from build123d import *

# Parameters (mm, degrees)
BOSS_EXTRUDE1_DEPTH           = 32
SKETCH1_3_R                   = 5
CUT_EXTRUDE1_DEPTH            = 94.618841069
CUT_EXTRUDE2_START            = -32
SKETCH2_R                     = 11.05
CUT_EXTRUDE2_DEPTH            = 5.5
M3_CLEARANCE_HOLE1_D          = 3.4
MOTOR_START                   = -5
MOTOR_POCKET_DEPTH            = 89.618841069
SKETCH6_R                     = 11
PILOT_DEPTH                   = 94.618841069
M3_CLEARANCE_HOLE2_D          = 3.4
SKETCH10_R                    = 10.35
BEARING_BORE_DEPTH            = 94.618841069
CUT_EXTRUDE6_START            = -12
CUT_EXTRUDE6_DEPTH            = 12
CUT_EXTRUDE14_START           = 3
CUT_EXTRUDE14_DEPTH           = 10
FILLET7_R                     = 5
FILLET11_R                    = 5
M3_CLEARANCE_HOLE4_D          = 3.4
CUT_EXTRUDE13_DEPTH           = 91.10972771
CUT_EXTRUDE13_DEPTH_BACK      = 3
SKETCH28_R                    = 4.7625
CUT_EXTRUDE17_DEPTH           = 45
SKETCH29_W                    = 30
SKETCH29_H                    = 10
CUT_EXTRUDE18_DEPTH           = 8.2625
CBORE_FOR_M3_SHCS1_AT_2_COUNT = 2
CBORE_FOR_M3_SHCS1_AT_2_PITCH = 25
CBORE_FOR_M3_SHCS1_AT_3_COUNT = 2
CBORE_FOR_M3_SHCS1_AT_3_PITCH = 32.015621187
CBORE_FOR_M3_SHCS1_AT_4_COUNT = 2
CBORE_FOR_M3_SHCS1_AT_4_PITCH = 20
SKETCH32_R                    = 3.25
CUT_EXTRUDE19_DEPTH           = 91.224649642


with BuildPart() as part:
    # Sketch1 → Boss-Extrude1 (new body)
    with BuildSketch(Plane(origin=(0, 0, 0), x_dir=(1, 0, 0), z_dir=(0, 1, 0))):
        with BuildLine():
            Line((0, 36.638737867), (40, -3.361262133))
            Line((40, -3.361262133), (40, -43.361262133))
            Line((40, -43.361262133), (39, -43.361262133))
            ThreePointArc((39, -43.361262133), (22.029437252, -50.390699384), (15, -67.361262133))
            Line((15, -67.361262133), (15, -78.361262133))
            Line((15, -78.361262133), (-15, -78.361262133))
            Line((-15, -78.361262133), (-15, -67.361262133))
            ThreePointArc((-15, -67.361262133), (-22.029437252, -50.390699384), (-39, -43.361262133))
            Line((-39, -43.361262133), (-40, -43.361262133))
            Line((-40, -43.361262133), (-40, -3.361262133))
            Line((-40, -3.361262133), (0, 36.638737867))
        make_face()
    extrude(amount=BOSS_EXTRUDE1_DEPTH)

    # Sketch1<3> → Cut-Extrude1 (cut, through all)
    with BuildSketch(Plane(origin=(0, 0, 0), x_dir=(1, 0, 0), z_dir=(0, 1, 0))):
        with Locations(Location((20, -30.981883618, 0), (0, 0, 270))):
            Circle(SKETCH1_3_R)
    extrude(amount=CUT_EXTRUDE1_DEPTH, mode=Mode.SUBTRACT)

    # Sketch2 → Cut-Extrude2 (cut)
    with BuildSketch(Plane(origin=(0, 32, 0), x_dir=(1, 0, 0), z_dir=(0, 1, 0)).offset(CUT_EXTRUDE2_START)):
        with Locations(Location((20, -30.981883618, 0), (0, 0, 90))):
            Circle(SKETCH2_R)
    extrude(amount=CUT_EXTRUDE2_DEPTH, mode=Mode.SUBTRACT)

    # M3 Clearance Hole1 (through all)
    with Locations(Plane(origin=(0, 32, 0), x_dir=(-1, 0, 0), z_dir=(0, 1, 0))):
        with Locations((-25.656854249, 25.325029368), (-25.656854249, 36.638737867), (-14.343145751, 36.638737867), (-14.343145751, 25.325029368)):
            Hole(M3_CLEARANCE_HOLE1_D / 2)

    # Sketch5 → Motor Pocket (cut, through all)
    with BuildSketch(Plane(origin=(0, 32, 0), x_dir=(1, 0, 0), z_dir=(0, 1, 0)).offset(MOTOR_START)):
        Polygon((0, 29.839906166), (-29.839906166, 0), (0, -29.839906166), (29.839906166, 0), align=None)
    extrude(amount=-MOTOR_POCKET_DEPTH, mode=Mode.SUBTRACT)

    # Sketch6 → Pilot (cut, through all)
    with BuildSketch(Plane(origin=(0, 32, 0), x_dir=(1, 0, 0), z_dir=(0, 1, 0))):
        with Locations(Location((0, 0, 0), (0, 0, 270))):
            Circle(SKETCH6_R)
    extrude(amount=-PILOT_DEPTH, mode=Mode.SUBTRACT)

    # M3 Clearance Hole2 (through all)
    with Locations(Plane(origin=(0, 32, 0), x_dir=(-1, 0, 0), z_dir=(0, 1, 0))):
        with Locations((21.9075, 0), (0, -21.9075), (-21.9075, 0), (0, 21.9075)):
            Hole(M3_CLEARANCE_HOLE2_D / 2)

    # Sketch10 → Bearing Bore (cut, through all)
    with BuildSketch(Plane(origin=(0, 32, 0), x_dir=(1, 0, 0), z_dir=(0, 1, 0))):
        with Locations(Location((-20, -30.981883618, 0), (0, 0, 270))):
            Circle(SKETCH10_R)
    extrude(amount=-BEARING_BORE_DEPTH, mode=Mode.SUBTRACT)

    # Sketch11 → Cut-Extrude6 (cut)
    with BuildSketch(Plane(origin=(0, 32, 0), x_dir=(1, 0, 0), z_dir=(0, 1, 0)).offset(CUT_EXTRUDE6_START)):
        with BuildLine():
            Line((-6, -32.361262133), (7, -32.361262133))
            ThreePointArc((7, -32.361262133), (12.052230702, -41.361462043), (22.05853806, -43.891767666))
            ThreePointArc((22.05853806, -43.891767666), (31.012194637, -43.049066482), (40, -43.361262133))
            Line((40, -43.361262133), (39, -43.361262133))
            ThreePointArc((39, -43.361262133), (22.029437252, -50.390699384), (15, -67.361262133))
            Line((15, -67.361262133), (15, -78.361262133))
            Line((15, -78.361262133), (-6, -78.361262133))
            Line((-6, -78.361262133), (-6, -32.361262133))
        make_face()
    extrude(amount=CUT_EXTRUDE6_DEPTH, mode=Mode.SUBTRACT)

    # Sketch26 → Cut-Extrude14 (cut)
    with BuildSketch(Plane(origin=(0, 20, 0), x_dir=(1, 0, 0), z_dir=(0, 1, 0)).offset(CUT_EXTRUDE14_START)):
        with BuildLine():
            Line((-6, -32.361262133), (-6.721452831, -32.361262133))
            ThreePointArc((-6.721452831, -32.361262133), (-11.061101946, -40.897457307), (-20, -44.331883618))
            Line((-20, -44.331883618), (-32.243689971, -44.331883618))
            ThreePointArc((-32.243689971, -44.331883618), (-19.788656467, -52.976399268), (-15, -67.361262133))
            Line((-15, -67.361262133), (-15, -78.361262133))
            Line((-15, -78.361262133), (-6, -78.361262133))
            Line((-6, -78.361262133), (-6, -32.361262133))
        make_face()
    extrude(amount=CUT_EXTRUDE14_DEPTH, mode=Mode.SUBTRACT)

    # Fillet7
    fillet7_edges = [part.edges().sort_by_distance(p)[0] for p in [
        (0, 16, -36.638737867),
    ]]
    fillet(fillet7_edges, radius=FILLET7_R)

    # Fillet11
    fillet11_edges = [part.edges().sort_by_distance(p)[0] for p in [
        (-40, 16, 3.361262133),
        (40, 16, 3.361262133),
    ]]
    fillet(fillet11_edges, radius=FILLET11_R)

    # M3 Clearance Hole4 (through all)
    with Locations(Plane(origin=(0, 20, 0), x_dir=(-1, 0, 0), z_dir=(0, 1, 0))):
        with Locations((0, 48.361262133), (0, 73.361262133)):
            Hole(M3_CLEARANCE_HOLE4_D / 2)

    # Sketch24 → Cut-Extrude13 (cut, two sides: drawn at the far end of the back side and taken through both)
    with BuildSketch(Plane.XZ.offset(-12.525).offset(-CUT_EXTRUDE13_DEPTH_BACK)):
        Polygon((1.558845727, 45.661262133), (3.117691454, 48.361262133), (1.558845727, 51.061262133), (-1.558845727, 51.061262133), (-3.117691454, 48.361262133), (-1.558845727, 45.661262133), align=None)
        Polygon((1.558845727, 70.661262133), (3.117691454, 73.361262133), (1.558845727, 76.061262133), (-1.558845727, 76.061262133), (-3.117691454, 73.361262133), (-1.558845727, 70.661262133), align=None)
    extrude(amount=CUT_EXTRUDE13_DEPTH + CUT_EXTRUDE13_DEPTH_BACK, mode=Mode.SUBTRACT)

    # Sketch28 → Cut-Extrude17 (cut)
    with BuildSketch(Plane.XY.offset(78.361262133)):
        with Locations((0, 7.7625)):
            Circle(SKETCH28_R)
    extrude(amount=-CUT_EXTRUDE17_DEPTH, mode=Mode.SUBTRACT)

    # Sketch29 → Cut-Extrude18 (cut)
    with BuildSketch(Plane.XZ):
        with Locations((0, 73.361262133)):
            Rectangle(SKETCH29_W, SKETCH29_H)
        with Locations((0, 48.361262133)):
            Rectangle(SKETCH29_W, SKETCH29_H)
    extrude(amount=-CUT_EXTRUDE18_DEPTH, mode=Mode.SUBTRACT)

    # Sketch30 → CBORE for M3 SHCS1 (revolve, cut)
    with BuildSketch(Plane(origin=(10, 20, 73.361262133), x_dir=(0, 0, 1), z_dir=(1, 0, 0))):
        Polygon((0, 0), (0, 20), (1.7, 20), (1.7, 3), (3.25, 3), (3.25, 0), align=None)
    cbore_for_m3_shcs1 = revolve(axis=Axis((10, 26.35, 73.361262133), (0, -1, 0)), mode=Mode.SUBTRACT)

    # CBORE for M3 SHCS1 at 2: CBORE for M3 SHCS1 ×2
    with Locations(*[(0, 0, -i * CBORE_FOR_M3_SHCS1_AT_2_PITCH) for i in range(1, CBORE_FOR_M3_SHCS1_AT_2_COUNT)]):
        add(cbore_for_m3_shcs1, mode=Mode.SUBTRACT)

    # CBORE for M3 SHCS1 at 3: CBORE for M3 SHCS1 ×2
    with Locations(*[Vector(-0.624695047554424, 0, -0.7808688094430305) * (i * CBORE_FOR_M3_SHCS1_AT_3_PITCH) for i in range(1, CBORE_FOR_M3_SHCS1_AT_3_COUNT)]):
        add(cbore_for_m3_shcs1, mode=Mode.SUBTRACT)

    # CBORE for M3 SHCS1 at 4: CBORE for M3 SHCS1 ×2
    with Locations(*[(-i * CBORE_FOR_M3_SHCS1_AT_4_PITCH, 0, 0) for i in range(1, CBORE_FOR_M3_SHCS1_AT_4_COUNT)]):
        add(cbore_for_m3_shcs1, mode=Mode.SUBTRACT)

    # Sketch32 → Cut-Extrude19 (cut, through all)
    with BuildSketch(Plane(origin=(0, 20, 0), x_dir=(1, 0, 0), z_dir=(0, 1, 0))):
        with Locations(Location((-10, -73.361262133, 0), (0, 0, 270))):
            Circle(SKETCH32_R)
        with Locations(Location((-10, -48.361262133, 0), (0, 0, 270))):
            Circle(SKETCH32_R)
    extrude(amount=CUT_EXTRUDE19_DEPTH, mode=Mode.SUBTRACT)


solid = part.part
The listing builds one solid part. Answer for the finished solid, in the listing's coordinates (mm). A direction names the side the tool comes from. Coordinates: 2 decimals unless noted, no trailing zeros. Write each loop counter-clockwise with the first axis right and the second up, starting at its lowest first coordinate (ties: lowest second). Pieces come first, ordered by that corner, then holes. Notation, with made-up numbers: M 45,1 L 91,1 A26 cw 91,27 Z; hole C -19.5,6 d11. An arc over 180 degrees is marked long. Use one line per item in the form item = value.
Item 1: Find section B-B, the plane z = 66. Give the vertices of the cut face in (x, y) (1 decimal).
Model answer:
outline = M -15,0 L 15,0 L 15,20 L -6,20 L -6,23 L -15,23 Z; hole C 0,7.8 d9.5
Item 2: Find the intervals of material crossed by probe 1 along Z at (x, y) = (0, 16.6); probe 2 along Z at (x, y) = (10, 15); probe 3 along Z at (x, y) = (6, 7), in increasing order.
Model answer:
probe_1 = -34.57 to -29.84, 29.84 to 46.66, 50.06 to 71.66, 75.06 to 78.36
probe_2 = -26.64 to -19.84, 19.84 to 46.66, 50.06 to 71.66, 75.06 to 78.36
probe_3 = -30.64 to -23.84, 23.84 to 43.36, 53.36 to 68.36
Item 3: Given P1, Ø3, axis at x = 2, y = 6, coming from the +Z side; P2, Ø10, axis at x = 30.5, y = 6, coming from the -Z side; P3, Ø5.5, axis at x = 0, z = -21.91, coming from the -Y side, each flat-ended and moving along its own axis, determine where each tip first touches the part or whether it passes through.
Model answer:
P1 = 33.36
P2 = -11.14
P3 = 27
Item 4: The mould has two halves that part along X. Classify faces 4 (the face through (9, 8.262, 75)), 5 (the face through (-2.35, 13.47, 72.03)), 6 (the face through (-21.84, 12.22, 50.58)), 7 (the face through (20.79, 15.78, -15.85)): released by +X, released by -X, zero draft, split by the parting line, or undercut.
Model answer:
face_4 = zero draft
face_5 = undercut
face_6 = released by -X
face_7 = released by +X
Item 5: Find section D-D, the plane z = 8. Give the vertices of the cut face in (x, y), plus the area to 3 significant figures.
Model answer:
outline = M -40,0 L -21.84,0 L -21.84,27 L -7.55,27 L -7.55,32 L -40,32 Z; M 7.55,27 L 21.84,27 L 21.84,0 L 40,0 L 40,32 L 7.55,32 Z
area = 1,310 mm2
Item 6: Find section A-A, the plane y = 21.5. Give the number of separate pieces and of enclosed holes in the cut face, plus the area to 3 significant figures.
Model answer:
separate_pieces = 1
enclosed_holes = 9
area = 2,760 mm2
Item 7: For faces 1 (the face through (11.4, 17, 72)), 2 (the face through (-6, 21, 56)), 3 (the face through (22, 5.5, 26)), determine the directions among +Z, -Z, +X, -X, +Y, -Y from which every point of the face is accessible in a straight line to the end or side of a thin tool.
Model answer:
face_1 = +Y
face_2 = +Z, +Y
face_3 = -Y
